The model under review builds one solid part; all positions refer to its coordinate system, in mm. Coordinates: 2 decimals unless noted, no trailing zeros. Order: outer loops, then holes, each group sorted by start corner. A loop starts at its lowest first (then second) coordinate and runs counter-clockwise, first axis right, second up.
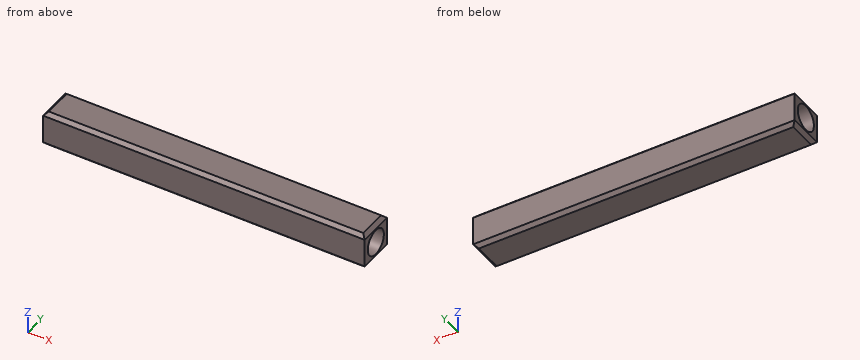
```python
from build123d import *

# Parameters (mm, degrees)
SKETCH1_W           = 22.5
SKETCH1_H           = 5
BOSS_EXTRUDE1_DEPTH = 5
SKETCH2_R           = 1.8
CUT_EXTRUDE1_DEPTH  = 5
CHAMFER1_SIZE       = 0.5


with BuildPart() as part:
    # Sketch1 → Boss-Extrude1 (new body)
    with BuildSketch(Plane.XY):
        with Locations((-11.25, 2.5)):
            Rectangle(SKETCH1_W, SKETCH1_H)
    boss_extrude1 = extrude(amount=BOSS_EXTRUDE1_DEPTH)

    # Sketch2 → Cut-Extrude1 (cut)
    with BuildSketch(Plane.ZY.offset(22.5)):
        with Locations((2.5, 2.5)):
            Circle(SKETCH2_R)
    cut_extrude1 = extrude(amount=-CUT_EXTRUDE1_DEPTH, mode=Mode.SUBTRACT)

    # Mirror1: Boss-Extrude1, Cut-Extrude1 across plane
    add(boss_extrude1.mirror(Plane(origin=(0, 0, 0), x_dir=(0, 0, 1), z_dir=(1, 0, 0))))
    add(cut_extrude1.mirror(Plane(origin=(0, 0, 0), x_dir=(0, 0, 1), z_dir=(1, 0, 0))), mode=Mode.SUBTRACT)

    # Chamfer1
    chamfer1_edges = [part.edges().sort_by_distance(p)[0] for p in [
        (0, 5, 5),
        (-22.5, 2.5, 5),
        (22.5, 2.5, 5),
        (22.5, 2.5, 0),
        (0, 0, 5),
        (-22.5, 2.5, 0),
        (0, 5, 0),
        (0, 0, 0),
    ]]
    chamfer(chamfer1_edges, length=CHAMFER1_SIZE)


solid = part.part
```
(1) We need section C-C, the plane x = 6. Write out the cut boundary in (y, z).
A:
outline: (0, 0.5) - (0.5, 0) - (4.5, 0) - (5, 0.5) - (5, 4.5) - (4.5, 5) - (0.5, 5) - (0, 4.5) - close
(2) For pin 1 Ø3 at (y, z) = (2.5, 2.5) entering from -X; pin 2 Ø1.8 at (y, z) = (2, 3) entering from +X, all flat-tipped, find the tip position at first contact; note any pin that passes through.
A:
pin 1: stops at x = -17.5
pin 2: stops at x = 17.5
(3) We need section A-A, the plane x = 18. Write out the cut boundary in (y, z), and give its area (3 significant figures).
A:
outline: (0, 0.5) - (0.5, 0) - (4.5, 0) - (5, 0.5) - (5, 4.5) - (4.5, 5) - (0.5, 5) - (0, 4.5) - close; hole circle Ø3.6 at (2.5, 2.5)
area: 14.3 mm2
(4) We need section B-B, the plane y = 2.5. Write out the cut boundary in (x, z).
A:
outline: (-22.5, 0.5) - (-22, 0) - (22, 0) - (22.5, 0.5) - (22.5, 0.7) - (17.5, 0.7) - (17.5, 4.3) - (22.5, 4.3) - (22.5, 4.5) - (22, 5) - (-22, 5) - (-22.5, 4.5) - (-22.5, 4.3) - (-17.5, 4.3) - (-17.5, 0.7) - (-22.5, 0.7) - close
(5) We need section D-D, the plane z = 2.5. Write out the cut boundary in (x, y), and give its area (3 significant figures).
A:
outline: (-22.5, 0) - (22.5, 0) - (22.5, 0.7) - (17.5, 0.7) - (17.5, 4.3) - (22.5, 4.3) - (22.5, 5) - (-22.5, 5) - (-22.5, 4.3) - (-17.5, 4.3) - (-17.5, 0.7) - (-22.5, 0.7) - close
area: 189 mm2
(6) Wall thickness on probe 1 along Y at (x, z) = (20.7, 2.5); probe 2 along X at (y, z) = (1.5, 3.25); probe 3 along Z at (x, y) = (18.5, 1): over which ranges is each line inside the solid? List them lowest first.
A:
probe 1: y = 0 to 0.7, 4.3 to 5
probe 2: x = -17.5 to 17.5
probe 3: z = 0 to 1.51, 3.49 to 5
